Autodesk Fusion 360 part; units mm, degrees
sketch "Sketch1" plane through (0, 0, 0) normal (0, 0, 1) x (1, 0, 0)
  circle A0 centre (0, 0) radius 45
  circle A1 centre (0, 0) radius 11
  circle A2 centre (0, 0) radius 4
  circle A3 centre (0, 0) radius 13.5
  line L0 (7.5056, 36) -> (3.7528, 42.5)
  line L1 (3.7528, 42.5) -> (-3.7528, 42.5)
  line L2 (-3.7528, 42.5) -> (-7.5056, 36)
  line L3 (-7.5056, 36) -> (-3.7528, 29.5)
  line L4 (-3.7528, 29.5) -> (3.7528, 29.5)
  line L5 (3.7528, 29.5) -> (7.5056, 36)
  line L6 (0, 0) -> (0, 29.5) construction
  circle A4 centre (0, 36) radius 9 construction
  line L7 (-13.3941, 1.6875) -> (-8.0282, 44.2781)
  line L8 (8.0282, 44.2781) -> (13.3941, 1.6875)
  point P0 (0, 36)
  dimension "d1" = 90
  dimension "d2" = 22
  dimension "d3" = 8
  dimension "d4" = 2.5
  dimension "d5" = 6.5
  dimension "d6" = 29.5
extrude "Extrude1" add sketch "Sketch1" along normal blind 8 contours A0 A3 L7 L8 | A3 picked at (0, 24.1667) makes body 1
pattern_circular "C-Pattern1" count 3 over 360 about axis through (0, 0, 1.75) along (0, 0, 1) of bodies 1 makes body 2 at (-20.0614, -11.8988, 0) makes body 3 at (20.3354, -11.4242, 0)
combine "Combine1" operation add target body 1 tool bodies 3 2
fillet "Fillet1" radius 12 3 edges at (12.6841, 7.3232, 4) (-12.6841, 7.3232, 4) (0, -14.6463, 4) on bodies 1
chamfer "Chamfer1" distance 0.5 angle 45 6 edges at (-8.0282, 44.2781, 4) (8.0282, 44.2781, 4) (42.36, -15.1864, 4) (-42.36, -15.1864, 4) (-34.3318, -29.0917, 4) (34.3318, -29.0917, 4) on bodies 1
For this review, take the finished solid that the model builds, in its own axes (mm). A direction names the side the tool comes from. Coordinates: 2 decimals unless noted, no trailing zeros. Loops run counter-clockwise (first coordinate to the right, second up) from the corner with the lowest first, then second, coordinate; pieces in that order, holes last. Notation, with made-up numbers: (23, 73) -> (65, 73) arc R20 ccw to (65, 80) -> close; hole circle Ø5 at (20.5, -2). An arc over 180 degrees is marked (long way). Return JSON: item names as keys, results as strings. Group by question number.
(1) Consider section D-D, the plane y = 27. Give the boundary of the cut face in (x, z), plus the area to 3 significant figures.
(2) Tool access review of faces 4 (the flat face through (5.66, 39.2, 3.94)), 5 (the flat face through (-19.058, -22.665, 3.944)), 6 (the flat face through (-29.51, -5.44, 3.94)): name each direction out of +Z, -Z, +X, -X, +Y, -Y from which nothing blocks a thin tool from reaching the whole face with its end or side.
(3) For pin 1 Ø3 at (x, z) = (23, 5) entering from +Y; pin 2 Ø17.5 at (x, y) = (0, 0) entering from +Z; pin 3 Ø1.5 at (y, z) = (2.5, 3.5) entering from -X; pin 4 Ø4 at (x, z) = (-31.5, 5.5) entering from +Y, all flat-tipped, find the tip position at first contact; note any pin that passes through.
(4) Consider section C-C, the plane z = 4.5. Count the separate pieces of the cut face and the enclosed holes in it, plus the area to 3 significant figures.
(5) Consider section B-B, the plane x = 0. Give the boundary of the cut face in (y, z).
(6) Mouldability with a two-part tool opening along X and no side actions: class faces 1 (the cylindrical face through (39.024, -22.408, 3.944)), 2 (the cylindrical face through (-38.92, -22.59, 3.94)), 3 (the flat face through (0, 42.5, 4)) as pulls with the +X half, pulls with the -X half, needs draft (parallel to the pull), parting line crosses it, or undercut.
(7) To check wall thickness, follow L1, parallel to Y at x = 0, z = 6.5; L2, parallel to X at y = -24, z = 4; L3, parallel to X at y = -13, z = 5.5. State the ranges of each line that lie inside material, in increasing order.
(8) Consider section A-A, the plane y = -2.5. Give the boundary of the cut face in (x, z).
Results below:
{
 "1": {"outline": "(-10.21, 0) -> (10.21, 0) -> (10.21, 8) -> (-10.21, 8) -> close", "area": "163 mm2"},
 "2": {"face 4": "+Z, -Z", "face 5": "+Z, -Z, -Y", "face 6": "+Z, -Z, -X, +Y"},
 "3": {"pin 1": "stops at y = 0.64", "pin 2": "passes through", "pin 3": "stops at x = -20.03", "pin 4": "stops at y = -5.43"},
 "4": {"separate pieces": "1", "enclosed holes": "4", "area": "1,790 mm2"},
 "5": {"outline": "(-15.67, 0) -> (-11, 0) -> (-11, 8) -> (-15.67, 8) -> close; (11, 0) -> (29.5, 0) -> (29.5, 8) -> (11, 8) -> close; (42.5, 0) -> (45, 0) -> (45, 8) -> (42.5, 8) -> close"},
 "6": {"face 1": "pulls with the +X half", "face 2": "pulls with the -X half", "face 3": "undercut"},
 "7": {"L1": "y = -15.67 to -11, 11 to 29.5, 42.5 to 45", "L2": "x = -38.07 to -35.22, -27.14 to -22.23, 22.23 to 27.14, 35.22 to 38.07", "L3": "x = -39.48 to -35.8, -26.56 to 26.56, 35.8 to 39.48"},
 "8": {"outline": "(-25.63, 0) -> (-10.71, 0) -> (-10.71, 8) -> (-25.63, 8) -> close; (10.71, 0) -> (25.63, 0) -> (25.63, 8) -> (10.71, 8) -> close"}
}
